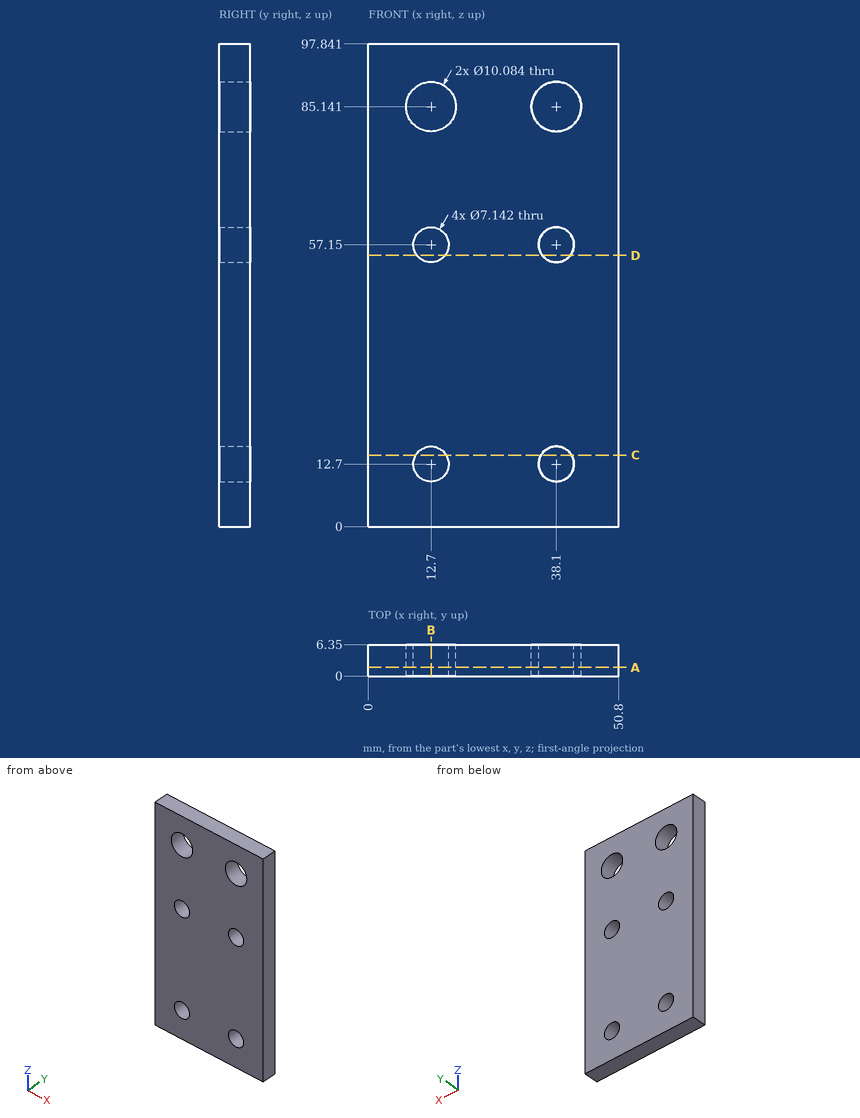
Geometry check sheet. Reference: drawing and pictorial views, mm from the part's lowest x, y, z. Give positions to 0.01 mm unless a question says otherwise; leave off trailing zeros. Order: outer loops, then holes, each group sorted by start corner. A loop starts at its lowest first (then second) coordinate and runs counter-clockwise, first axis right, second up. Notation, with made-up numbers: M 62.25,42 L 89.25,42 A20 ccw 89.25,71 Z; hole C -25.5,74.5 d7. An arc over 180 degrees is marked long. Answer as a JSON object with one key per item and string values. Group by question number.
1) Cross-section at B-B (x = 12.7). Enter the section's corners in (y, z).
2) Cross-section at D-D (z = 55). Enter the section's corners in (x, y).
3) Cross-section at A-A (y = 1.75). Enter the section's corners in (x, z).
4) Cross-section at C-C (z = 14.5). Give the number of separate pieces and of enclosed holes in the cut face, then the cut area to 3 significant figures.
5) Scan lines: line 1 along X through (y, z) = (2, 12.7); line 2 along Z through (x, y) = (38.1, 2.25); line 3 along Z through (x, y) = (37.5, 5.75) (1 decimal). Record each from-to range of solid material in increasing order. Write a range as [from, to].
Result sheet:
{
 "1": {"outline": "M 0,0 L 6.35,0 L 6.35,9.13 L 0,9.13 Z; M 0,16.27 L 6.35,16.27 L 6.35,53.58 L 0,53.58 Z; M 0,60.72 L 6.35,60.72 L 6.35,80.1 L 0,80.1 Z; M 0,90.18 L 6.35,90.18 L 6.35,97.84 L 0,97.84 Z"},
 "2": {"outline": "M 0,0 L 9.85,0 L 9.85,6.35 L 0,6.35 Z; M 15.55,0 L 35.25,0 L 35.25,6.35 L 15.55,6.35 Z; M 40.95,0 L 50.8,0 L 50.8,6.35 L 40.95,6.35 Z"},
 "3": {"outline": "M 0,0 L 50.8,0 L 50.8,97.84 L 0,97.84 Z; hole C 12.7,85.14 d10.08; hole C 12.7,12.7 d7.14; hole C 12.7,57.15 d7.14; hole C 38.1,85.14 d10.08; hole C 38.1,12.7 d7.14; hole C 38.1,57.15 d7.14"},
 "4": {"separate pieces": "3", "enclosed holes": "0", "area": "244 mm2"},
 "5": {"line 1": "x = [0, 9.13], [16.27, 34.53], [41.67, 50.8]", "line 2": "z = [0, 9.13], [16.27, 53.58], [60.72, 80.1], [90.18, 97.84]", "line 3": "z = [0, 9.2], [16.2, 53.6], [60.7, 80.1], [90.1, 97.8]"}
}
